Autodesk Inventor part; units mm, degrees
ref_plane "YZ Plane" through (0, 0, 0) normal (1, 0, 0) x (0, 1, 0)
ref_plane "XZ Plane" through (0, 0, 0) normal (0, 1, 0) x (-1, 0, 0)
ref_plane "XY Plane" through (0, 0, 0) normal (0, 0, 1) x (1, 0, 0)
sketch "Sketch1" plane through (0, 0, 0) normal (0, 0, 1) x (1, 0, 0)
  line L0 (-35.56, 0) -> (35.56, 0)
  line L1 (0, -71.12) -> (0, 71.12)
  line L2 (-25.4, 50.8) -> (25.4, 50.8)
  line L3 (25.4, 50.8) -> (25.4, -50.8)
  line L4 (25.4, -50.8) -> (-25.4, -50.8)
  line L5 (-25.4, -50.8) -> (-25.4, 50.8)
  point P0 (0, 0)
  point P1 (-25.4, 0)
  point P2 (0, 50.8)
  dimension "d0" = 101.6
  dimension "d1" = 50.8
extrude "Extrusion1" add sketch "Sketch1" along normal mid plane 9.525
sketch "Sketch2" plane through (25.4, -50.8, 4.7625) normal (1, 0, 0) x (0, 0, -1)
  point P0 (4.7625, 50.8)
  point P1 (4.7625, 76.2)
  point P2 (4.7625, 50.8)
  point P3 (4.7625, 25.4)
  dimension "d4" = 25.4
  dimension "d5" = 25.4
hole "Hole1" at (25.4, 25.4, 0) at (25.4, 0, 0) at (25.4, -25.4, 0) direction (-1, 0, 0) diameter 3.683 depth 19.05 tip angle 118
mirror "Mirror1" about plane through (0, 0, 0) normal (1, 0, 0) of "Hole1"
properties part number "plate_connect_block"
The listing builds one solid part. Answer for the finished solid, in the listing's coordinates (mm). A direction names the side the tool comes from. Round coordinates to 2 decimals unless told otherwise and drop trailing zeros. Write each loop counter-clockwise with the first axis right and the second up, starting at its lowest first coordinate (ties: lowest second). Pieces come first, ordered by that corner, then holes. Notation, with made-up numbers: (50.25, 69.5) -> (63.25, 69.5) arc R29 ccw to (63.25, 95.5) -> close; hole circle Ø3 at (14, -33.75). An arc over 180 degrees is marked (long way). Answer as a JSON object with one key per item and string values. Group by question number.
Q1. Determine the mould class of faces 1 (the face through (-5.436, -25.67, -0.172)), 2 (the face through (0, 50.8, 0)), 3 (the face through (15.742, 27.198, 0.399)), 4 (the face through (0, 1, -4.762)) for opening direction Y: pulls with the +Y half, pulls with the -Y half, needs draft (parallel to the pull), parting line crosses it, or undercut.
Q2. Straight lines are drawn through the part: line 1 along Y through (x, z) = (-15.75, 0); line 2 along Z through (x, y) = (-21, -25.4). For each, find the intervals that lie inside material, in ascending order.
Q3. Which of the six approach directions +Z, -Z, +X, -X, +Y, -Y give full straight-line access (tool end or side, diameter ignored) to faces 5 (the face through (-25.4, -1, -2)), 6 (the face through (15.742, -23.602, 0.399)), 7 (the face through (-15.742, 23.602, 0.399))?
Q4. Section A-A (x = -9.5) is taken. Write down the section's boundary in (y, z).
Q5. Each of these flat-tipped pins is pushed along its axis until it touches: pin 1 Ø2 at (y, z) = (25.4, 0) entering from +X; pin 2 Ø3 at (y, z) = (-25.4, 0) entering from +X; pin 3 Ø2 at (y, z) = (0, 0) entering from -X. Where does it stop, or does it pass through?
Check values:
{
 "1": {"face 1": "undercut", "face 2": "pulls with the +Y half", "face 3": "undercut", "face 4": "needs draft"},
 "2": {"line 1": "-50.8 to -27.24, -23.56 to -1.84, 1.84 to 23.56, 27.24 to 50.8", "line 2": "-4.76 to -1.84, 1.84 to 4.76"},
 "3": {"face 5": "+Z, -Z, -X, +Y, -Y", "face 6": "+X", "face 7": "-X"},
 "4": {"outline": "(-50.8, -4.76) -> (50.8, -4.76) -> (50.8, 4.76) -> (-50.8, 4.76) -> close; hole circle Ø3.68 at (-25.4, 0); hole circle Ø3.68 at (0, 0); hole circle Ø3.68 at (25.4, 0)"},
 "5": {"pin 1": "x = 5.84", "pin 2": "x = 6.14", "pin 3": "x = -5.84"}
}
